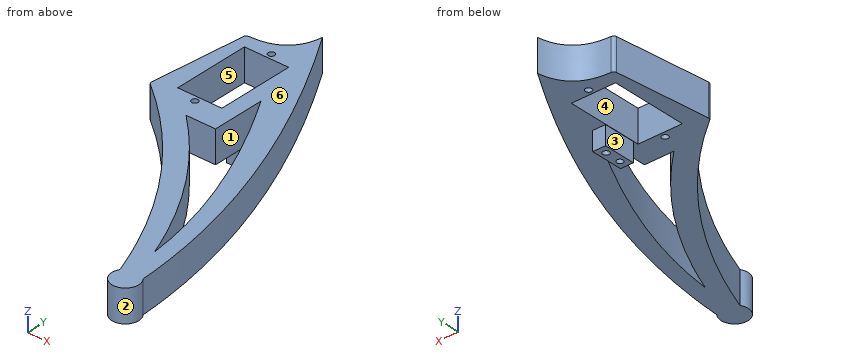
```python
from build123d import *

# Parameters (mm, degrees)
CYLINDER020_R     = 1
CYLINDER020_DEPTH = 10
CYLINDER019_R     = 1
CYLINDER019_DEPTH = 10
BOX008_W          = 4
BOX008_H          = 10
BOX008_DEPTH      = 8.9
SKETCH003_W       = 13.8
SKETCH003_H       = 24
SKETCH003_R       = 1
EXTRUDE003_DEPTH  = 10
FILLET001_R       = 1


with BuildPart() as cylinder020:
    # Cylinder020 → Cylinder020 (new body)
    with BuildSketch(Plane(origin=(9, -2.9, -11.7), x_dir=(1, 0, 0), z_dir=(0, 0, 1))):
        Circle(CYLINDER020_R)
    extrude(amount=CYLINDER020_DEPTH)


with BuildPart() as cylinder019:
    # Cylinder019 → Cylinder019 (new body)
    with BuildSketch(Plane(origin=(9, -7.9, -11.7), x_dir=(1, 0, 0), z_dir=(0, 0, 1))):
        Circle(CYLINDER019_R)
    extrude(amount=CYLINDER019_DEPTH)


with BuildPart() as cube:
    # Box008 → Box008 (new body)
    with BuildSketch(Plane(origin=(7, -10.4, -5.9), x_dir=(1, 0, 0), z_dir=(0, 0, 1))):
        with Locations((2, 5)):
            Rectangle(BOX008_W, BOX008_H)
    extrude(amount=BOX008_DEPTH)


with BuildPart() as version_final:
    # Sketch003 → Extrude003 (new body)
    with BuildSketch(Plane.XY):
        with BuildLine():
            Line((-10, 16.128428), (-13.297334, -14.6392))
            add(Edge.make_bspline(
                [(-13.297334, -14.6392), (20.347338, -40.345566), (35.627229, -81.672969)],
                knots=[0, 0, 0, 1, 1, 1], degree=2))
            ThreePointArc((35.627229, -81.672969), (39.484607, -88.059425), (42.451137, -81.213558))
            add(Edge.make_bspline(
                [(4.23934, 27.2126), (39.721497, -30.208815), (42.451137, -81.213558)],
                knots=[0, 0, 0, 1, 1, 1], degree=2))
            add(Edge.make_bspline(
                [(-10, 16.128428), (2.6632, 16.087), (4.23934, 27.2126)],
                knots=[0, 0, 0, 1, 1, 1], degree=2))
        make_face()
        Rectangle(SKETCH003_W, SKETCH003_H, mode=Mode.SUBTRACT)
        with Locations((0, -13.75)):
            Circle(SKETCH003_R, mode=Mode.SUBTRACT)
        with Locations((0, 13.75)):
            Circle(SKETCH003_R, mode=Mode.SUBTRACT)
        with BuildLine():
            add(Edge.make_bspline(
                [(2.569153, -19.891897), (25.299458, -40.964581), (36.64809, -70.471016)],
                knots=[0, 0, 0, 1, 1, 1], degree=2))
            add(Edge.make_bspline(
                [(36.64809, -70.471016), (33.5686, -40), (11.784026, -3.578896)],
                knots=[0, 0, 0, 1, 1, 1], degree=2))
            Line((11.784026, -3.578896), (11.784026, -19.891897))
            Line((11.784026, -19.891897), (2.569153, -19.891897))
        make_face(mode=Mode.SUBTRACT)
    extrude(amount=EXTRUDE003_DEPTH)

    # Fillet001
    fillet001_edges = [version_final.edges().sort_by_distance(p)[0] for p in [
        (-10, 16.128428, 5),
        (-13.297334, -14.6392, 5),
    ]]
    fillet(fillet001_edges, radius=FILLET001_R)

    # Fusion012: union Cube
    add(cube.part)

    # Cut006: cut Cylinder019
    add(cylinder019.part, mode=Mode.SUBTRACT)

    # Cut007: cut Cylinder020
    add(cylinder020.part, mode=Mode.SUBTRACT)


solid = version_final.part
```
Design review of the part built by this model. Coordinates are the model's own, in mm. Face numbers are marked on the shaded views. A direction names the side the tool comes from. Round coordinates to 2 decimals unless told otherwise and drop trailing zeros. Write each loop counter-clockwise with the first axis right and the second up, starting at its lowest first coordinate (ties: lowest second). Pieces come first, ordered by that corner, then holes. Notation, with made-up numbers: (71, 25.25) -> (79, 25.25) arc R18 cw to (79, 45.25) -> close; hole circle Ø3 at (66, 77). An arc over 180 degrees is marked (long way). Answer in a Markdown table with one row per item.
Q1. To check wall thickness, follow L1, parallel to Y at x = 9, z = -4; L2, parallel to Y at x = 5.5, z = 5.5; L3, parallel to X at y = -2.9, z = -4.65. State the ranges of each line that lie inside material, in increasing order. Write a range as [from, to].
The answers:
| item | result |
|---|---|
| L1 | [-10.4, -8.9], [-6.9, -3.9], [-1.9, -0.4] |
| L2 | [-31.75, -22.69], [-19.89, -12], [12, 25.16] |
| L3 | [7, 8], [10, 11] |
Q2. Take a section at B-B, the plane z = 1.5. Count the separate pieces of the cut face and the enclosed holes in it, then the cut area to 3 significant figures.
The answers:
| item | result |
|---|---|
| separate pieces | 1 |
| enclosed holes | 4 |
| area | 1,600 mm² |
Q3. Clearance check with flat-ended pins moving along their axes: pin 1 Ø5 at (x, z) = (10, 5.5) entering from -Y; pin 2 Ø1 at (y, z) = (-30, 6) entering from -X; pin 3 Ø1.2 at (x, y) = (9, -2.9) entering from -Z; pin 4 Ø1.2 at (x, y) = (0, 13.75) entering from +Z. State where each tip first meets the part, or that it passes through.
The answers:
| item | result |
|---|---|
| pin 1 | y = -39.96 |
| pin 2 | x = 3.38 |
| pin 3 | z = -1.7 |
| pin 4 | through |
Q4. Take a section at A-A, the plane z = -3.5. State the section outline as (x, y) points, then the cut area to 3 significant figures.
The answers:
| item | result |
|---|---|
| outline | (7, -10.4) -> (11, -10.4) -> (11, -0.4) -> (7, -0.4) -> close; hole circle Ø2 at (9, -7.9); hole circle Ø2 at (9, -2.9) |
| area | 33.7 mm² |
Q5. For the marked faces 5 and 6, list the 3-axis set-ups (+Z, -Z, +X, -X, +Y, -Y) from which the entire face can be reached by the end or side of a thin tool; tool diameter is ignored.
The answers:
| item | result |
|---|---|
| face 5 | +Z, -Z |
| face 6 | +Z, +X, -X, +Y, -Y |
Q6. Draft analysis for pull direction X (two halves, no side actions). For the marked faces 1, 2, 3 and 4, state which applies: +X half, -X half, draft (parallel to the pull), parting line (faces both ways), or undercut.
The answers:
| item | result |
|---|---|
| face 1 | undercut |
| face 2 | parting line |
| face 3 | -X half |
| face 4 | undercut |
